Here's the drawing with two shaded views (mm, measured from the low corner). I have some questions. Coordinates: 2 decimals unless noted, no trailing zeros. Order: outer loops, then holes, each group sorted by start corner. A loop starts at its lowest first (then second) coordinate and runs counter-clockwise, first axis right, second up. Notation, with made-up numbers: M 80.25,-13.75 L 90.25,-13.75 A7 ccw 90.25,-5.75 Z; hole C 10.25,46.5 d7. An arc over 180 degrees is marked long. Put each result on its own line as item: value. Start each with the question number.
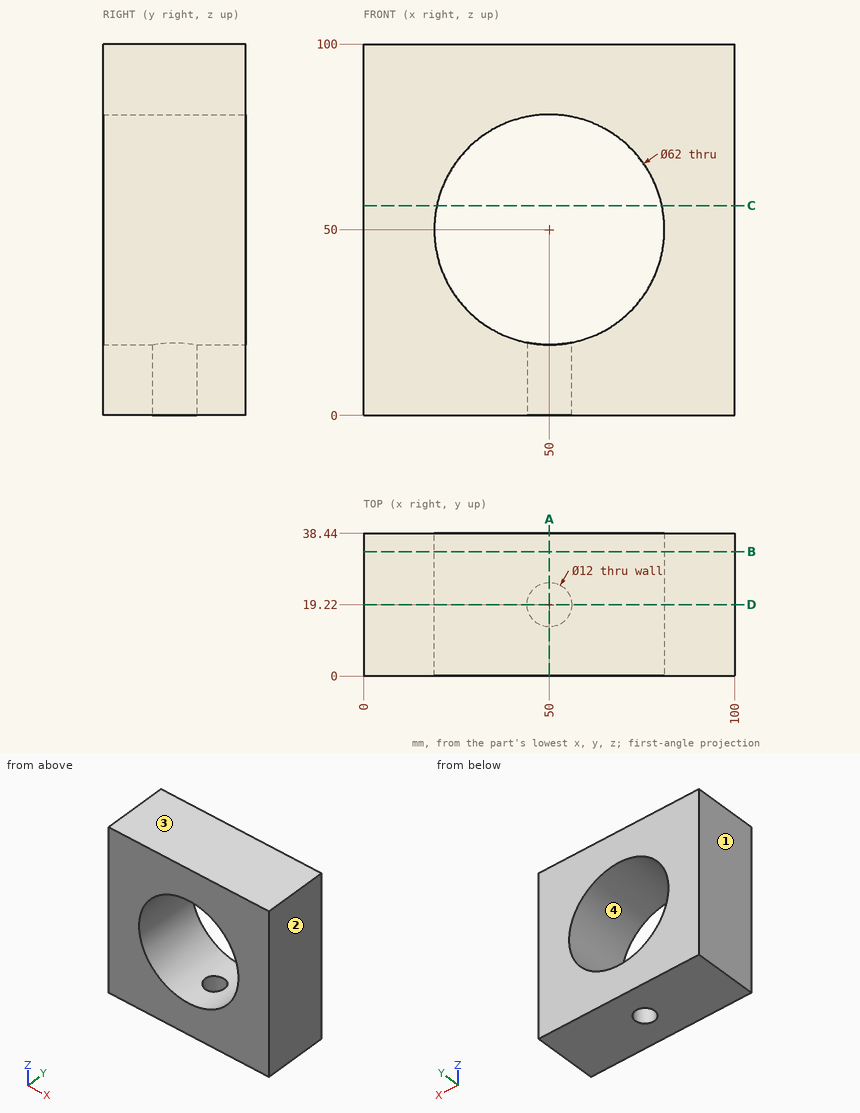
Item 1: I need wall thicknesses on probe 1 along X at (y, z) = (19, 8); probe 2 along Z at (x, y) = (50, 11); probe 3 along X at (y, z) = (26, 48.5). Which ranges of each line are inside material? Lowest first, please.
Item 2: If we section it at C-C on z = 56.5: Write out the boundary of the cut face in (x, y), then the cut area to 3 significant figures.
Item 3: For pin 1 Ø7 at (x, y) = (50, 19.22) entering from -Z; pin 2 Ø2 at (y, z) = (8.5, 34) entering from -X, each with a flat end and sliding along its axis, tell me the tip position at first contact or that it passes through.
Item 4: If we section it at D-D on y = 19.22: Write out the boundary of the cut face in (x, z).
Item 5: If we section it at B-B on y = 33.5: Write out the boundary of the cut face in (x, z), then the cut area to 3 significant figures.
Item 6: If we mould it in two halves opening along X, with no side actions, what happens to the marked faces 1, 2, 3 and 4? For each: released by +X, released by -X, zero draft, split by the parting line, or undercut.
Item 7: If we section it at A-A on x = 50: Write out the boundary of the cut face in (y, z).
Geometry check:
1. probe 1: x = 0 to 44, 56 to 100
1. probe 2: z = 0 to 19, 81 to 100
1. probe 3: x = 0 to 19.04, 80.96 to 100
2. outline: M 0,0 L 19.69,0 L 19.69,38.44 L 0,38.44 Z; M 80.31,0 L 100,0 L 100,38.44 L 80.31,38.44 Z
2. area: 1,510 mm²
3. pin 1: stops at z = 80.8
3. pin 2: stops at x = 0
4. outline: M 0,0 L 44,0 L 44,19.59 A31 cw long 56,19.59 L 56,0 L 100,0 L 100,100 L 0,100 Z
5. outline: M 0,0 L 100,0 L 100,100 L 0,100 Z; hole C 50,50 d62
5. area: 6,980 mm²
6. face 1: released by -X
6. face 2: released by +X
6. face 3: zero draft
6. face 4: undercut
7. outline: M 0,0 L 13.22,0 L 13.22,19 L 0,19 Z; M 0,81 L 38.44,81 L 38.44,100 L 0,100 Z; M 25.22,0 L 38.44,0 L 38.44,19 L 25.22,19 Z
